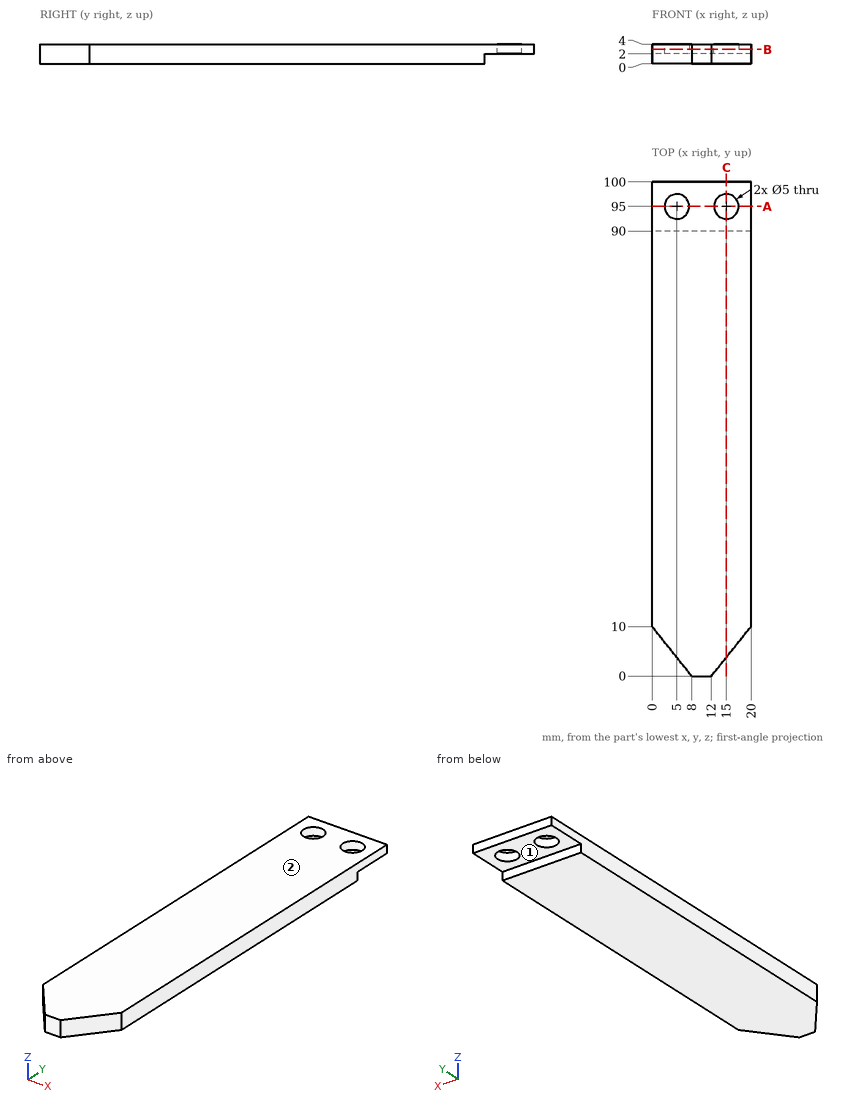
Verification items for this drawing (mm, ordinates from the low corner). A direction names the side the tool comes from. Coordinates: 2 decimals unless noted, no trailing zeros. Order: outer loops, then holes, each group sorted by start corner. A loop starts at its lowest first (then second) coordinate and runs counter-clockwise, first axis right, second up. Notation, with made-up numbers: (30, -5.5) -> (70, -5.5) arc R20 ccw to (70, 12.5) -> close; hole circle Ø8 at (27, -13). An arc over 180 degrees is marked (long way). Answer as CSV lines item,"result". Start each with the question number.
1) Set-up check for the marked faces 1 and 2: record each of +Z, -Z, +X, -X, +Y, -Y from which the full face is reachable in a straight line by a thin tool's end or side.
2) Gauge pin test, flat ends, axial feed: pin 1 Ø3 at (x, y) = (12.5, 95.5) entering from -Z; pin 2 Ø3 at (x, y) = (5, 95) entering from +Z. Record the tip position at first contact, or that the pin passes through.
3) Material ranges on L1, parallel to Y at x = 9.25, z = 0.35; L2, parallel to Y at x = 15, z = 3, recorded low to high. Write a range as [from, to].
4) Cross-section at A-A, the plane y = 95. Record the boundary of the cut face in (x, z).
5) Cross-section at C-C, the plane x = 15. Record the boundary of the cut face in (y, z).
6) Cross-section at B-B, the plane z = 2.9. Record the boundary of the cut face in (x, y), then the cut area to 3 significant figures.
Conclusion:
1,face 1,"-Z, +X, -X, +Y"
1,face 2,"+Z, +X, -X, +Y, -Y"
2,pin 1,"stops at z = 2"
2,pin 2,"passes through"
3,L1,"y = [0, 90]"
3,L2,"y = [3.75, 92.5], [97.5, 100]"
4,outline,"(0, 2) -> (2.5, 2) -> (2.5, 4) -> (0, 4) -> close; (7.5, 2) -> (12.5, 2) -> (12.5, 4) -> (7.5, 4) -> close; (17.5, 2) -> (20, 2) -> (20, 4) -> (17.5, 4) -> close"
5,outline,"(3.75, 0) -> (90, 0) -> (90, 2) -> (92.5, 2) -> (92.5, 4) -> (3.75, 4) -> close; (97.5, 2) -> (100, 2) -> (100, 4) -> (97.5, 4) -> close"
6,outline,"(0, 10) -> (8, 0) -> (12, 0) -> (20, 10) -> (20, 100) -> (0, 100) -> close; hole circle Ø5 at (5, 95); hole circle Ø5 at (15, 95)"
6,area,"1,880 mm²"
